from build123d import *

# Parameters (mm, degrees)
SHORT_LEVER_DEPTH      = 1.8
SHORT_LEVER_DEPTH_BACK = 1.8
LEVER_CUT_DEPTH        = 4.04793
FILLET_1_R             = 0.7


with BuildPart() as part:
    # Short → Short_Lever (new, two sides: drawn at the far end of the back side and taken through both)
    with BuildSketch(Plane(origin=(2.85, 0, 0), x_dir=(0, 0, -1), z_dir=(1, 0, 0)).offset(-SHORT_LEVER_DEPTH_BACK)):
        with BuildLine():
            Line((5.55, 4.85), (5.55, 6.042820323))
            ThreePointArc((5.55, 6.042820323), (5.431703238, 6.365779512), (5.132789449, 6.535918596))
            Line((5.132789449, 6.535918596), (-8.65, 8.85))
            Line((-8.65, 8.85), (-8.625163165, 8.997929482))
            Line((-8.625163165, 8.997929482), (5.157626284, 6.683848078))
            ThreePointArc((5.157626284, 6.683848078), (5.54621421, 6.462667269), (5.7, 6.042820323))
            Line((5.7, 6.042820323), (5.7, 4.85))
            Line((5.7, 4.85), (5.55, 4.85))
        make_face()
    extrude(amount=SHORT_LEVER_DEPTH + SHORT_LEVER_DEPTH_BACK)

    # Эскиз2 → Lever_Cut (cut)
    with BuildSketch(Plane(origin=(0, 4.95, 0), x_dir=(1, 0, 0), z_dir=(0, 1, 0))):
        Polygon((1.05, 5.157626284), (1.35, -8.65), (1.05, -8.65), align=None)
        Polygon((4.65, 5.157626284), (4.65, -8.65), (4.35, -8.65), align=None)
        with BuildLine():
            Line((2.35, 5.8), (3.35, 5.8))
            Line((3.35, 5.8), (3.20551955, -1.905624011))
            ThreePointArc((3.20551955, -1.905624011), (3.115706509, -2.11411119), (2.90557227, -2.2))
            Line((2.90557227, -2.2), (2.79442773, -2.2))
            ThreePointArc((2.79442773, -2.2), (2.584293491, -2.11411119), (2.49448045, -1.905624011))
            Line((2.49448045, -1.905624011), (2.35, 5.8))
        make_face()
    extrude(amount=LEVER_CUT_DEPTH, mode=Mode.SUBTRACT)

    # Скругление1
    fillet_1_edges = [part.edges().sort_by_distance(p)[0] for p in [
        (1.349730184, 8.923964741, 8.637581583),
        (4.350269816, 8.923964741, 8.637581583),
    ]]
    fillet(fillet_1_edges, radius=FILLET_1_R)


solid = part.part
The listing builds one solid part. Answer for the finished solid, in the listing's coordinates (mm). A direction names the side the tool comes from. Give positions to 0.01 mm unless a question says otherwise; leave off trailing zeros. Write each loop counter-clockwise with the first axis right and the second up, starting at its lowest first coordinate (ties: lowest second). Pieces come first, ordered by that corner, then holes.
1) Section A-A (z = -3.5) is taken. Write down the section's boundary in (x, y), and give its area (3 significant figures).
2) Given P1, Ø1, axis at x = 2, y = 5, coming from the +Z side, flat-ended and moving along its own axis, determine where the tip first touches the part or whether it passes through.
3) Find the intervals of material crossed by L1, parallel to Z at x = 2.05, y = 5.9; L2, parallel to Y at x = 1.7, z = -4.25, in increasing order.
4) Section C-C (y = 5.2) is taken. Write down the section's boundary in (x, z), and give its area (3 significant figures).
5) Section D-D (z = 5) is taken. Write down the section's boundary in (x, y).
6) A tool of negligible diameter and unlimited length cuts with its end or side. For faces 1 (the face through (2, 5, -5.55)), 2 (the face through (2, 5, -5.7)), from which of +Z, -Z, +X, -X, +Y, -Y can it reach the whole face along a straight path? Write none if from no direction.
7) Section B-B (x = 2.2) is taken. Write down the section's boundary in (y, z).
Response:
1. outline: (1.09, 6.81) - (2.39, 6.81) - (2.39, 6.96) - (1.09, 6.96) - close; (3.31, 6.81) - (4.61, 6.81) - (4.61, 6.96) - (3.31, 6.96) - close
1. area: 0.398 mm2
2. P1: stops at z = -5.55
3. L1: z = -5.7 to -5.55
3. L2: y = 6.68 to 6.84
4. outline: (1.05, -5.7) - (2.35, -5.7) - (2.35, -5.55) - (1.05, -5.55) - close; (3.35, -5.7) - (4.65, -5.7) - (4.65, -5.55) - (3.35, -5.55) - close
4. area: 0.391 mm2
5. outline: (1.27, 8.24) - (4.43, 8.24) - (4.43, 8.39) - (1.27, 8.39) - close
6. face 1: +Z, +X, -X, -Y
6. face 2: -Z, +X, -X, +Y, -Y
7. outline: (4.85, -5.7) - (6.04, -5.7) arc R0.65 ccw to (6.68, -5.16) - (9, 8.63) - (8.85, 8.65) - (6.54, -5.13) arc R0.5 cw to (6.04, -5.55) - (4.85, -5.55) - close
